from build123d import *

# Parameters (mm, degrees)
SKETCH_1_R      = 1.6
EXTRUDE_1_DEPTH = 2


with BuildPart() as part:
    # 草图1 → 凸台-拉伸1 (new body)
    with BuildSketch(Plane.XY):
        with BuildLine():
            Line((0, -28), (58, -28))
            ThreePointArc((58, -28), (59.414213562, -27.414213562), (60, -26))
            Line((60, -26), (60, 24))
            ThreePointArc((60, 24), (59.414213562, 25.414213562), (58, 26))
            Line((58, 26), (0, 26))
            ThreePointArc((0, 26), (-1.414213562, 25.414213562), (-2, 24))
            Line((-2, 24), (-2, -26))
            ThreePointArc((-2, -26), (-1.414213562, -27.414213562), (0, -28))
        make_face()
        with Locations((5, 23)):
            Circle(SKETCH_1_R, mode=Mode.SUBTRACT)
        with Locations((55, 23)):
            Circle(SKETCH_1_R, mode=Mode.SUBTRACT)
        with Locations((55, -23)):
            Circle(SKETCH_1_R, mode=Mode.SUBTRACT)
        with Locations((5, -23)):
            Circle(SKETCH_1_R, mode=Mode.SUBTRACT)
        with BuildLine():
            Line((9, 13), (9, -13))
            ThreePointArc((9, -13), (6, -16), (3, -13))
            Line((3, -13), (3, 13))
            ThreePointArc((3, 13), (6, 16), (9, 13))
        make_face(mode=Mode.SUBTRACT)
        with BuildLine():
            Line((18, 13), (18, -13))
            ThreePointArc((18, -13), (15, -16), (12, -13))
            Line((12, -13), (12, 13))
            ThreePointArc((12, 13), (15, 16), (18, 13))
        make_face(mode=Mode.SUBTRACT)
        with BuildLine():
            Line((27, 13), (27, -13))
            ThreePointArc((27, -13), (24, -16), (21, -13))
            Line((21, -13), (21, 13))
            ThreePointArc((21, 13), (24, 16), (27, 13))
        make_face(mode=Mode.SUBTRACT)
        with BuildLine():
            Line((36, 13), (36, -13))
            ThreePointArc((36, -13), (33, -16), (30, -13))
            Line((30, -13), (30, 13))
            ThreePointArc((30, 13), (33, 16), (36, 13))
        make_face(mode=Mode.SUBTRACT)
        with BuildLine():
            Line((45, 13), (45, -13))
            ThreePointArc((45, -13), (42, -16), (39, -13))
            Line((39, -13), (39, 13))
            ThreePointArc((39, 13), (42, 16), (45, 13))
        make_face(mode=Mode.SUBTRACT)
        with BuildLine():
            Line((54, 13), (54, -13))
            ThreePointArc((54, -13), (51, -16), (48, -13))
            Line((48, -13), (48, 13))
            ThreePointArc((48, 13), (51, 16), (54, 13))
        make_face(mode=Mode.SUBTRACT)
    extrude(amount=EXTRUDE_1_DEPTH)


solid = part.part
Design review of the part built by this model. Coordinates are the model's own, in mm. A direction names the side the tool comes from. Coordinates: 2 decimals unless noted, no trailing zeros. Order: outer loops, then holes, each group sorted by start corner. A loop starts at its lowest first (then second) coordinate and runs counter-clockwise, first axis right, second up.
Item 1: Take a section at D-D, the plane y = 7. Write out the cut boundary in (x, z).
Item 2: Take a section at A-A, the plane x = 24. Write out the cut boundary in (y, z).
Item 3: The part is to be moulded in two halves that separate along X. For faces 1 (the flat face through (9, 0, 1)), 2 (the flat face through (-2, -1, 1)), 3 (the flat face through (29, -28, 1)), say which applies: pulls with the +X half, pulls with the -X half, needs draft (parallel to the pull), parting line crosses it, or undercut.
Item 4: Take a section at B-B, the plane y = 23. Write out the cut boundary in (x, z).
Item 5: For line 1 (Y direction, x = 55, z = 1.5); line 2 (Y direction, x = 4.5, z = 1.3); line 3 (Y direction, x = 5.5, z = 0.65), list the stretches that pass through material, from the lowest coordinate up.
Item 6: Take a section at C-C, the plane x = 55. Write out the cut boundary in (y, z), then the cut area to 3 significant figures.
Item 7: For faces 4 (the cylindrical face through (42, -16, 1)), 5 (the cylindrical face through (-1.43, -27.4, 0.99)), list the 3-axis set-ups (+Z, -Z, +X, -X, +Y, -Y) from which the entire face can be reached by the end or side of a thin tool; tool diameter is ignored.
The answers:
1. outline: (-2, 0) - (3, 0) - (3, 2) - (-2, 2) - close; (9, 0) - (12, 0) - (12, 2) - (9, 2) - close; (18, 0) - (21, 0) - (21, 2) - (18, 2) - close; (27, 0) - (30, 0) - (30, 2) - (27, 2) - close; (36, 0) - (39, 0) - (39, 2) - (36, 2) - close; (45, 0) - (48, 0) - (48, 2) - (45, 2) - close; (54, 0) - (60, 0) - (60, 2) - (54, 2) - close
2. outline: (-28, 0) - (-16, 0) - (-16, 2) - (-28, 2) - close; (16, 0) - (26, 0) - (26, 2) - (16, 2) - close
3. face 1: undercut
3. face 2: pulls with the -X half
3. face 3: needs draft
4. outline: (-2, 0) - (3.4, 0) - (3.4, 2) - (-2, 2) - close; (6.6, 0) - (53.4, 0) - (53.4, 2) - (6.6, 2) - close; (56.6, 0) - (60, 0) - (60, 2) - (56.6, 2) - close
5. line 1: y = -28 to -24.6, -21.4 to 21.4, 24.6 to 26
5. line 2: y = -28 to -24.52, -21.48 to -15.6, 15.6 to 21.48, 24.52 to 26
5. line 3: y = -28 to -24.52, -21.48 to -15.96, 15.96 to 21.48, 24.52 to 26
6. outline: (-28, 0) - (-24.6, 0) - (-24.6, 2) - (-28, 2) - close; (-21.4, 0) - (21.4, 0) - (21.4, 2) - (-21.4, 2) - close; (24.6, 0) - (26, 0) - (26, 2) - (24.6, 2) - close
6. area: 95.2 mm2
7. face 4: +Z, -Z
7. face 5: +Z, -Z, -X, -Y
